Geometry: see drawing. Coordinates: mm, zero at the bounding-box minimum. A direction names the side the tool comes from. Round coordinates to 2 decimals unless told otherwise and drop trailing zeros. Loops run counter-clockwise (first coordinate to the right, second up) from the corner with the lowest first, then second, coordinate; pieces in that order, holes last. Notation, with made-up numbers: (66.5, -6) - (123.5, -6) arc R22 ccw to (123.5, 6) - close; hole circle Ø5 at (-27.75, 1.25). An arc over 180 degrees is marked (long way). Answer in a Markdown table with one row per item. Add a question column.
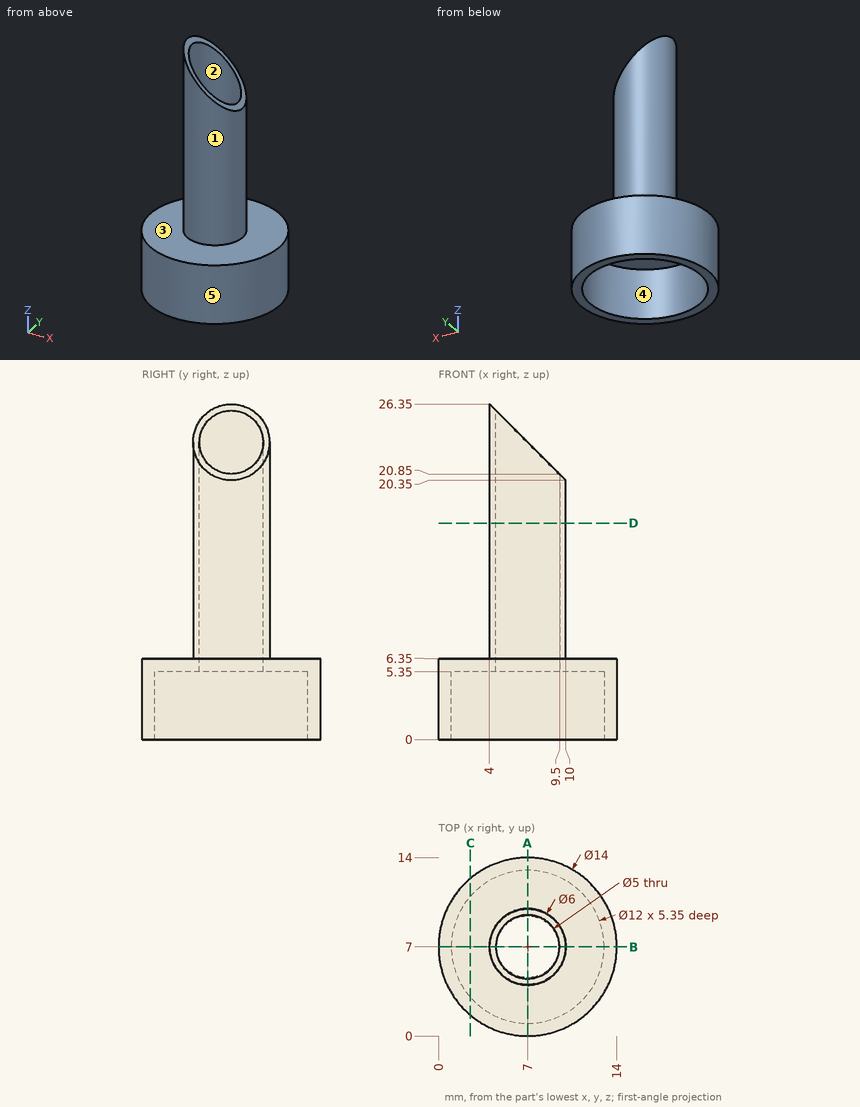
1) Contact query for flat-ended pins moving along their axis: pin 1 Ø5 at (y, z) = (11, 5) entering from -X; pin 2 Ø4 at (x, y) = (7, 7) entering from +Z; pin 3 Ø1.5 at (y, z) = (4, 23) entering from -X; pin 4 Ø5 at (x, z) = (12.5, 3.5) entering from +Y. Output: stop coordinate, or through.
2) Reachability of the marked faces 1 and 2 from +Z, -Z, +X, -X, +Y, -Y: full face, straight path, thin tool, end or side. Return the list, or none.
3) Section C-C, the plane x = 2.5. Return the cut outline in (y, z).
4) Section B-B, the plane y = 7. Return the cut outline in (x, z), and give its area (3 significant figures).
5) Pull-direction query (Y, two-part tool) for the marked faces 3, 4 and 5; classes: pulls with the +Y half, pulls with the -Y half, needs draft (parallel to the pull), parting line crosses it, or undercut.
6) Material intervals for line 1 along Y through (x, z) = (7, 13); line 2 along Y through (x, z) = (7, 1.6), sorted ascending. Write a range as from..to.
7) Section A-A, the plane x = 7. Return the cut outline in (y, z), and give its area (3 significant figures).
8) Section D-D, the plane z = 17. Return the cut outline in (x, y), and give its area (3 significant figures).
Evaluation:
| question | item | result |
|---|---|---|
| 1 | pin 1 | stops at x = 0.16 |
| 1 | pin 2 | passes through |
| 1 | pin 3 | stops at x = 5.02 |
| 1 | pin 4 | stops at y = 13.32 |
| 2 | face 1 | +Z |
| 2 | face 2 | +Z, -Z |
| 3 | outline | (1.64, 0) - (3.03, 0) - (3.03, 5.35) - (10.97, 5.35) - (10.97, 0) - (12.36, 0) - (12.36, 6.35) - (1.64, 6.35) - close |
| 4 | outline | (0, 0) - (1, 0) - (1, 5.35) - (4.5, 5.35) - (4.5, 25.85) - (4, 26.35) - (4, 6.35) - (0, 6.35) - close; (9.5, 5.35) - (13, 5.35) - (13, 0) - (14, 0) - (14, 6.35) - (10, 6.35) - (10, 20.35) - (9.5, 20.85) - close |
| 4 | area | 36.7 mm² |
| 5 | face 3 | needs draft |
| 5 | face 4 | undercut |
| 5 | face 5 | parting line crosses it |
| 6 | line 1 | y = 4..4.5, 9.5..10 |
| 6 | line 2 | y = 0..1, 13..14 |
| 7 | outline | (0, 0) - (1, 0) - (1, 5.35) - (4.5, 5.35) - (4.5, 23.35) - (4, 23.35) - (4, 6.35) - (0, 6.35) - close; (9.5, 5.35) - (13, 5.35) - (13, 0) - (14, 0) - (14, 6.35) - (10, 6.35) - (10, 23.35) - (9.5, 23.35) - close |
| 7 | area | 36.7 mm² |
| 8 | outline | circle Ø6 at (7, 7); hole circle Ø5 at (7, 7) |
| 8 | area | 8.64 mm² |
